Can you work these out from the model? Positions are in its coordinate system, mm. Give positions to 0.01 mm unless a question says otherwise; leave off trailing zeros. Order: outer loops, then holes, each group sorted by start corner. A loop starts at its lowest first (then second) coordinate and runs counter-clockwise, first axis right, second up. Notation, with made-up numbers: (45.5, -13.5) - (65.5, -13.5) arc R25 cw to (65.5, 24.5) - close; hole circle Ø8 at (18, 28.25). An arc over 180 degrees is marked (long way). One line per question, with ' | ' between items.
Autodesk Inventor part; units mm, degrees
ref_plane "YZ Plane" through (0, 0, 0) normal (1, 0, 0) x (0, 1, 0)
ref_plane "XZ Plane" through (0, 0, 0) normal (0, 1, 0) x (-1, 0, 0)
ref_plane "XY Plane" through (0, 0, 0) normal (0, 0, 1) x (1, 0, 0)
sketch "Esquisse1" plane through (0, 0, 0) normal (0, 1, 0) x (-1, 0, 0)
  line L0 (0, 0) -> (8, 0)
  line L1 (8, 0) -> (8, -60.5)
  line L2 (8, -60.5) -> (0, -60.5)
  line L3 (0, -60.5) -> (0, 0)
  circle A0 centre (4, -4) radius 1.5
  circle A1 centre (4, -56.5) radius 1.5
  dimension "d1" = 8
  dimension "d2" = 3
  dimension "d3" = 4
  dimension "d4" = 4
  dimension "d5" = 4
  dimension "d6" = 4
  dimension "d7" = 3
  dimension "d11" = 52.5
extrude "Extrusion1" add sketch "Esquisse1" along normal blind 5
fillet "Congé1" radius 4 4 edges at (-8, 2.5, 0) (0, 2.5, 0) (0, 2.5, -60.5) (-8, 2.5, -60.5)
equation "\"d3\" = 0.5 * d1"
equation "\"d4\" = d3"
equation "\"d5\" = d3"
equation "\"d6\" = d5"
equation "\"d7\" = d2"
properties part number "biellette1" material "Acier inoxydable"
(1) If we mould it in two halves opening along X, with no side actions, what happens to faces 1 (the face through (0, 2, -31)), 2 (the face through (-8, 2, -30)), 3 (the face through (-4.806, 2.465, -57.765)), 4 (the face through (-4, 0, -30))? For each: released by +X, released by -X, zero draft, split by the parting line, or undercut.
Answer below:
face 1: released by +X | face 2: released by -X | face 3: undercut | face 4: zero draft
(2) Imagine slicing it at A-A (y = 2.2). Count the separate pieces of the cut face and the enclosed holes in it, and give its area (3 significant figures).
Answer below:
separate pieces: 1 | enclosed holes: 2 | area: 456 mm^2
(3) Imagine slicing it at D-D (x = -1). List the corners of the cut face in (y, z) for me, and give its area (3 significant figures).
Answer below:
outline: (0, -59.15) - (5, -59.15) - (5, -1.35) - (0, -1.35) - close | area: 289 mm^2
(4) Imagine slicing it at B-B (x = -3.5). List the corners of the cut face in (y, z) for me.
Answer below:
outline: (0, -60.47) - (5, -60.47) - (5, -57.91) - (0, -57.91) - close; (0, -55.09) - (5, -55.09) - (5, -5.41) - (0, -5.41) - close; (0, -2.59) - (5, -2.59) - (5, -0.03) - (0, -0.03) - close
(5) Will these pins go through, and if not, where does the flat tip stop? pin 1 (1 mm diameter, centred on x = -6, y = 2.5, fed in from -Z); pin 2 (1.5 mm diameter, centred on x = -3, y = 4, fed in from -Z).
Answer below:
pin 1: z = -60.21 | pin 2: z = -60.49
(6) Imagine slicing it at C-C (x = -6.5). List the corners of the cut face in (y, z) for me, and give its area (3 significant figures).
Answer below:
outline: (0, -59.62) - (5, -59.62) - (5, -0.88) - (0, -0.88) - close | area: 294 mm^2
(7) If I drill on line 1 (Z direction, x = -4, y = 1.6); line 2 (Z direction, x = -5.25, y = 1.75); line 3 (X direction, y = 2.9, z = -56), over which ranges is the centre line in solid material (lowest first)?
Answer below:
line 1: -60.5 to -58, -55 to -5.5, -2.5 to 0 | line 2: -60.3 to -57.33, -55.67 to -4.83, -3.17 to -0.2 | line 3: -8 to -5.41, -2.59 to 0
